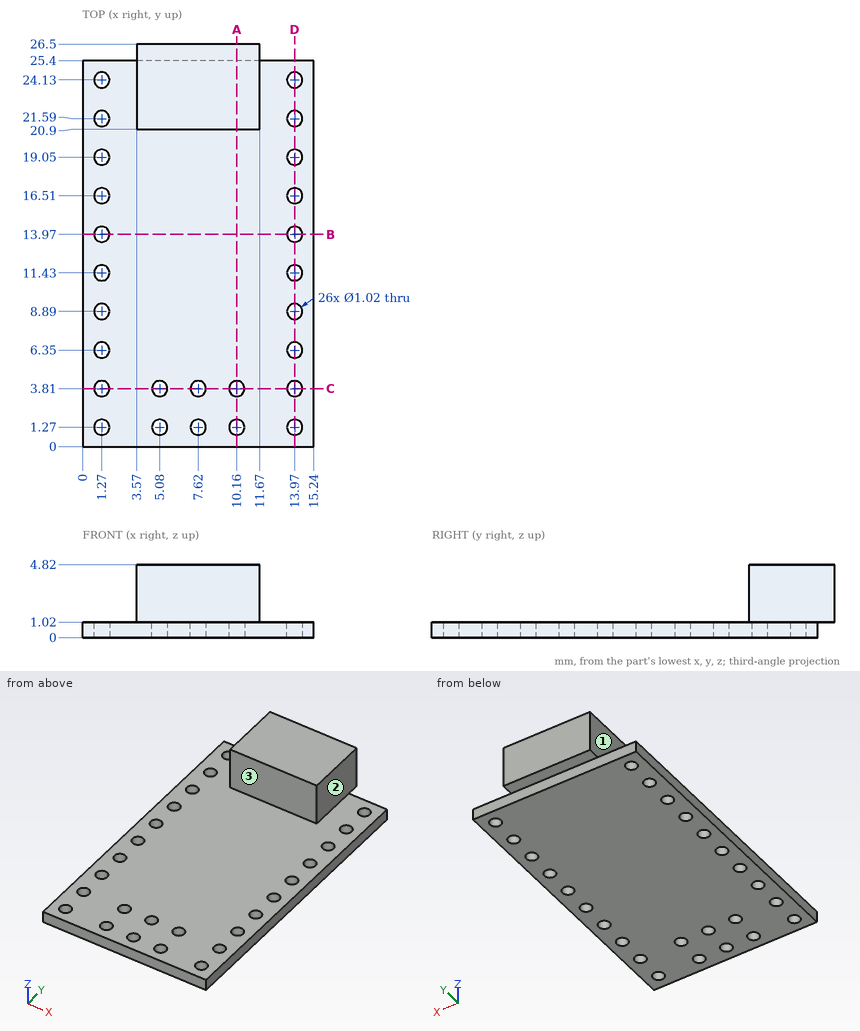
Print and shaded views of the part. All mm, measured from the part's lowest x, y and z. A direction names the side the tool comes from. Round coordinates to 2 decimals unless told otherwise and drop trailing zeros. Write each loop counter-clockwise with the first axis right and the second up, starting at its lowest first coordinate (ties: lowest second). Pieces come first, ordered by that corner, then holes. Notation, with made-up numbers: (50, -40) -> (106, -40) arc R23 ccw to (106, -16) -> close; hole circle Ø11 at (72.25, -22). An arc over 180 degrees is marked (long way). Answer in a Markdown table with one row per item. Add a question column.
Item 1: Which spindle directions (+Z, -Z, +X, -X, +Y, -Y) get a long thin tool onto all of the face, cutting with end or side? Do the marked faces 1, 2 and 3. Say none if no direction does.
Item 2: Saw through at D-D, the plane x = 13.97. Count the separate pieces of the cut face and the enclosed holes in it, then the cut area to 3 significant figures.
Item 3: Drop flat-ended pins along their axis: pin 1 Ø1.1 at (y, z) = (23, 2) entering from +X; pin 2 Ø2 at (y, z) = (23.5, 3) entering from -X; pin 3 Ø0.9 at (x, y) = (1.27, 8.89) entering from -Z; pin 4 Ø1.3 at (x, y) = (13.97, 11.43) entering from +Z. Give the stop position or say it passes through.
Item 4: Saw through at C-C, the plane y = 3.81. Write the cut outline in (x, z), then the cut area to 3 significant figures.
Item 5: Saw through at B-B, the plane y = 13.97. Write the cut outline in (x, z).
Item 6: Drill centre lines: line 1 (Z direction, x = 12.5, y = 11.75); line 2 (Y direction, x = 9.75, z = 2.5); line 3 (X direction, y = 25, z = 1.1). Where is each one in solid material? Low to high. Write a range as from..to.
Item 7: Saw through at A-A, the plane x = 10.16. Write the cut outline in (y, z).
Findings below:
| question | item | result |
|---|---|---|
| 1 | face 1 | +Z, -X, +Y, -Y |
| 1 | face 2 | +Z, +X, +Y, -Y |
| 1 | face 3 | +Z, +X, -X, -Y |
| 2 | separate pieces | 11 |
| 2 | enclosed holes | 0 |
| 2 | area | 15.5 mm^2 |
| 3 | pin 1 | stops at x = 11.67 |
| 3 | pin 2 | stops at x = 3.57 |
| 3 | pin 3 | passes through |
| 3 | pin 4 | stops at z = 1.02 |
| 4 | outline | (0, 0) -> (0.76, 0) -> (0.76, 1.02) -> (0, 1.02) -> close; (1.78, 0) -> (4.57, 0) -> (4.57, 1.02) -> (1.78, 1.02) -> close; (5.59, 0) -> (7.11, 0) -> (7.11, 1.02) -> (5.59, 1.02) -> close; (8.13, 0) -> (9.65, 0) -> (9.65, 1.02) -> (8.13, 1.02) -> close; (10.67, 0) -> (13.46, 0) -> (13.46, 1.02) -> (10.67, 1.02) -> close; (14.48, 0) -> (15.24, 0) -> (15.24, 1.02) -> (14.48, 1.02) -> close |
| 4 | area | 10.3 mm^2 |
| 5 | outline | (0, 0) -> (0.76, 0) -> (0.76, 1.02) -> (0, 1.02) -> close; (1.78, 0) -> (13.46, 0) -> (13.46, 1.02) -> (1.78, 1.02) -> close; (14.48, 0) -> (15.24, 0) -> (15.24, 1.02) -> (14.48, 1.02) -> close |
| 6 | line 1 | z = 0..1.02 |
| 6 | line 2 | y = 20.9..26.5 |
| 6 | line 3 | x = 3.57..11.67 |
| 7 | outline | (0, 0) -> (0.76, 0) -> (0.76, 1.02) -> (0, 1.02) -> close; (1.78, 0) -> (3.3, 0) -> (3.3, 1.02) -> (1.78, 1.02) -> close; (4.32, 0) -> (25.4, 0) -> (25.4, 1.02) -> (26.5, 1.02) -> (26.5, 4.82) -> (20.9, 4.82) -> (20.9, 1.02) -> (4.32, 1.02) -> close |
